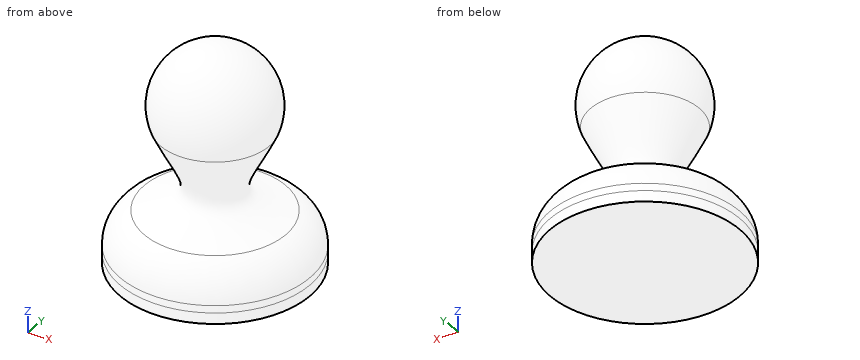
```python
from build123d import *

# Parameters (mm, degrees)
F2_R     = 5.25
F3_DEPTH = 3.5
F4_R     = 13
F5_DEPTH = 1.5


with BuildPart() as f1:
    # F0 (on Front) → F1 (revolve)
    with BuildSketch(Plane.XZ):
        with BuildLine():
            Line((-13, 0), (0, 0))
            Line((0, 0), (0, 28))
            ThreePointArc((0, 28), (-6.6208594363, 24.4904588101), (-7.4326741465, 17.0410550813))
            add(Edge.make_bspline(
                [(-7.4326741465, 17.0410550813), (-5.1480043112, 12.0772723951), (-1.8048124165, 8.1672623986), (-7.1835572352, 6.6008977536), (-9.6816832971, 5.7087090893)],
                knots=[0, 0, 0, 0, 0.495820355, 0.8469277652, 0.8469277652, 0.8469277652, 0.8469277652], degree=3))
            ThreePointArc((-9.6816832971, 5.7087090893), (-12.0870782037, 3.8802416144), (-13, 1))
            Line((-13, 1), (-13, 0))
        make_face()
    revolve(axis=Axis((0, 0, 14), (0, 0, 1)))

    # F2 (on face) → F3 (cut)
    with BuildSketch(Plane(origin=(0, 0, 0), x_dir=(1, 0, 0), z_dir=(0, 0, -1))):
        with Locations((-5.6291651246, -3.25)):
            Circle(F2_R)
        with Locations((5.6291651246, -3.25)):
            Circle(F2_R)
        with Locations((0, 6.5)):
            Circle(F2_R)
    extrude(amount=-F3_DEPTH, mode=Mode.SUBTRACT)

    # F4 (on face) → F5 (join)
    with BuildSketch(Plane(origin=(0, 0, 0), x_dir=(1, 0, 0), z_dir=(0, 0, -1))):
        Circle(F4_R)
    extrude(amount=F5_DEPTH)


solid = f1.part
```
Here's how the part is built. I have some questions about the finished solid (model axes, mm). Coordinates: 2 decimals unless noted, no trailing zeros. Order: outer loops, then holes, each group sorted by start corner. A loop starts at its lowest first (then second) coordinate and runs counter-clockwise, first axis right, second up.
1) Imagine slicing it at A-A on y = -6.5. State how many separate pieces and enclosed holes the cut face has, and give its area (3 significant figures).
2) I need wall thicknesses on line 1 (X direction, y = 3.25, z = 2.5); line 2 (Z direction, x = 6.5, y = -1.75); line 3 (Z direction, x = -1, y = -6). Which ranges of each line are inside material? Lowest first, please.
3) Imagine slicing it at C-C on z = 5. List the corners of the cut face in (x, y) for me.
4) Will these pins go through, and if not, where does the flat tip stop? pin 1 (2 mm diameter, centred on x = -5, y = -9, fed in from +Z); pin 2 (12 mm diameter, centred on y = -6, z = 23, fed in from +X); pin 3 (5 mm diameter, centred on x = 4, y = 4, fed in from +Z).
Response values:
1. separate pieces: 2
1. enclosed holes: 1
1. area: 195 mm2
2. line 1: x = -12.35 to -10.88, -0.38 to 0.38, 10.88 to 12.35
2. line 2: z = -1.5 to 0, 3.5 to 6.77, 15.57 to 24.32
2. line 3: z = -1.5 to 0, 3.5 to 7.03, 14.29 to 25.2
3. outline: circle Ø22 at (0, 0)
4. pin 1: stops at z = 5.85
4. pin 2: stops at x = 7.97
4. pin 3: stops at z = 27.35
